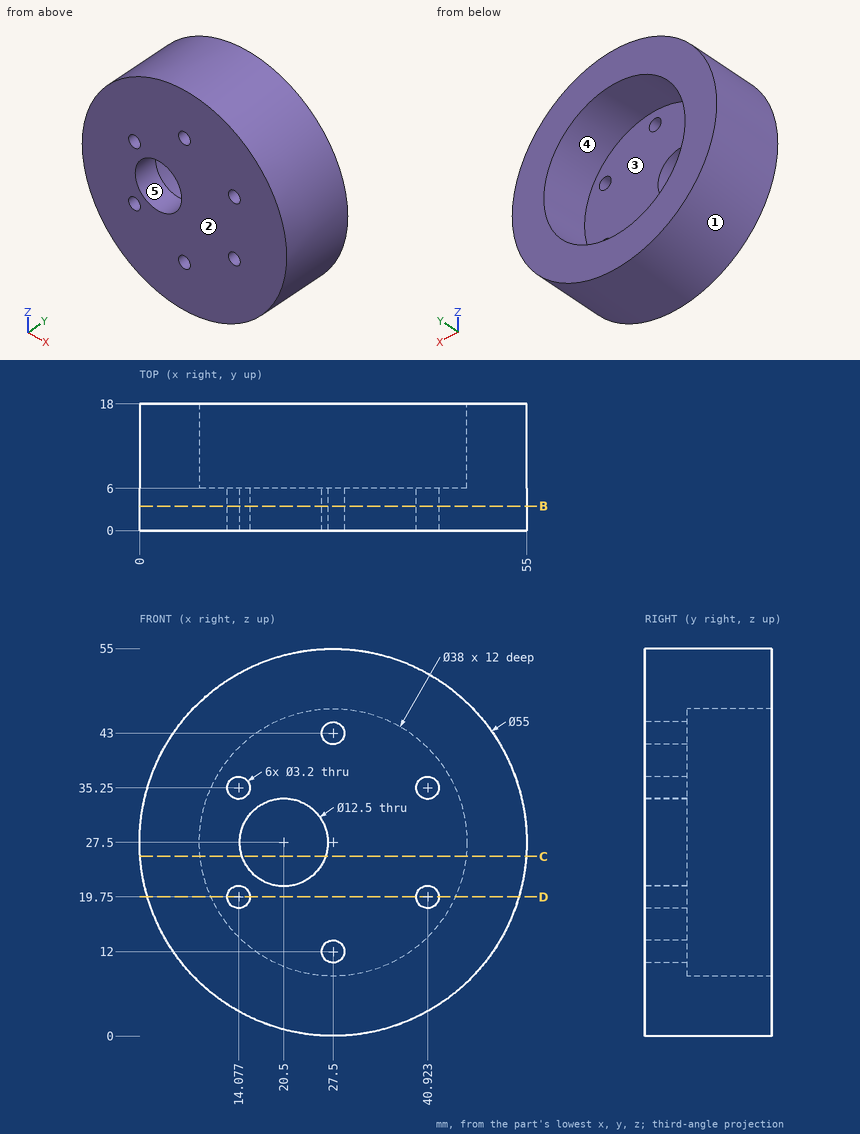
Check sheet for the drawn part. Datum: minimum x, y, z corner. Units: mm. A direction names the side the tool comes from. Round coordinates to 2 decimals unless told otherwise and drop trailing zeros. Write each loop counter-clockwise with the first axis right and the second up, starting at its lowest first coordinate (ties: lowest second). Pieces come first, ordered by that corner, then holes. Notation, with made-up numbers: (45.5, -26) - (104.5, -26) arc R27 cw to (104.5, 8) - close; hole circle Ø11 at (77.25, -13.75). An arc over 180 degrees is marked (long way). Return JSON: item names as keys, results as strings.
Q1. Cross-section at C-C (z = 25.5). Record the boundary of the cut face in (x, y) (1 decimal), then the cut area to 3 significant figures.
Returned:
{"outline": "(0.1, 0) - (14.6, 0) - (14.6, 6) - (8.6, 6) - (8.6, 18) - (0.1, 18) - close; (26.4, 0) - (54.9, 0) - (54.9, 18) - (46.4, 18) - (46.4, 6) - (26.4, 6) - close", "area": "463 mm²"}
Q2. Depth check by flat-ended pin: P1, Ø10, axis at y = 15, z = 8, coming from the -X side; P2, Ø8, axis at y = 11.5, z = 47.5, coming from the -X side (1 decimal); P3, Ø1.5, axis at y = 6, z = 14.5, coming from the +X side. Enter the tip coordinate at first touch or a pass-through.
Returned:
{"P1": "stops at x = 4.13", "P2": "stops at x = 5.1", "P3": "stops at x = 52.12"}
Q3. Cross-section at D-D (z = 19.75). Record the boundary of the cut face in (x, y) (1 decimal).
Returned:
{"outline": "(1.1, 0) - (12.5, 0) - (12.5, 6) - (10.2, 6) - (10.2, 18) - (1.1, 18) - close; (15.7, 0) - (39.3, 0) - (39.3, 6) - (15.7, 6) - close; (42.5, 0) - (53.9, 0) - (53.9, 18) - (44.8, 18) - (44.8, 6) - (42.5, 6) - close"}
Q4. Draft check along X on the marked faces 1, 2 and 3. Enter one of: released by +X, released by -X, zero draft, split by the parting line, or undercut.
Returned:
{"face 1": "split by the parting line", "face 2": "zero draft", "face 3": "undercut"}
Q5. Scan lines: L1, parallel to Y at x = 37.5, z = 20.5; L2, parallel to Z at x = 41, y = 12.5; L3, parallel to X at y = 10.25, z = 18.5 (1 decimal). Record each from-to range of solid material in increasing order. Write a range as from..to.
Returned:
{"L1": "y = 0..6", "L2": "z = 3.54..14.13, 40.87..51.46", "L3": "x = 1.5..10.8, 44.2..53.5"}
Q6. Cross-section at B-B (y = 3.5). Record the boundary of the cut face in (x, z), then the cut area to 4 significant figures.
Returned:
{"outline": "circle Ø55 at (27.5, 27.5); hole circle Ø3.2 at (14.08, 19.75); hole circle Ø3.2 at (14.08, 35.25); hole circle Ø12.5 at (20.5, 27.5); hole circle Ø3.2 at (27.5, 12); hole circle Ø3.2 at (27.5, 43); hole circle Ø3.2 at (40.92, 19.75); hole circle Ø3.2 at (40.92, 35.25)", "area": "2,205 mm²"}
Q7. Access from +Z, -Z, +X, -X, +Y, -Y to the whole of each face (thin tool, end or side, straight path). Record for the marked faces 4 and 5.
Returned:
{"face 4": "+Y", "face 5": "+Y, -Y"}
